```python
from build123d import *

# Parameters (mm, degrees)
ENCLOSURE_SHELL_SKETCH_W      = 76
ENCLOSURE_SHELL_SKETCH_H      = 54
ENCLOSURE_SHELL_FEATURE_DEPTH = 32
ENCLOSURE_GAP_SKETCH_W        = 73
ENCLOSURE_GAP_SKETCH_H        = 51
ENCLOSURE_GAP_FEATURE_DEPTH   = 30
CAMERA_CORD_HOLE_SKETCH_W     = 20
CAMERA_CORD_HOLE_SKETCH_H     = 12
CAMERA_CORD_HOLE_DEPTH        = 3
BATTERY_CUT_REACH             = 78
BATTERY_CUT_DIRECTION_2_DEPTH = 1
RIGHT_TAB_FEATURE_SKETCH_W    = 8
RIGHT_TAB_FEATURE_SKETCH_H    = 5
RIGHT_TAB_FEATURE_DEPTH       = 25
LEFT_TAB_FEATURE_SKETCH_W     = 8
LEFT_TAB_FEATURE_SKETCH_H     = 5
LEFT_TAB_FEATURE_DEPTH        = 25
SKETCH1_W                     = 76
SKETCH1_H                     = 54
BOSS_EXTRUDE1_DEPTH           = 20
CUT_EXTRUDE2_START            = -2
SKETCH5_W                     = 72
SKETCH5_H                     = 50
CUT_EXTRUDE2_DEPTH            = 18
SCREW_SHELL_SKETCH_R          = 2.5
SCREW_SHELL_FEATURE_DEPTH     = 1
SKETCH6_W                     = 58
SKETCH6_H                     = 38
CUT_EXTRUDE3_DEPTH            = 2
SCREW_HOLE_SKETCH_R           = 1.6
CUT_EXTRUDE4_DEPTH            = 2
FILLET1_R                     = 3
FILLET2_R                     = 3
FILLET3_R                     = 3
FILLET4_R                     = 3


with BuildPart() as part:
    # Enclosure Shell Sketch → Enclosure Shell Feature (new body)
    with BuildSketch(Plane(origin=(0, 0, 0), x_dir=(1, 0, 0), z_dir=(0, 1, 0))):
        Rectangle(ENCLOSURE_SHELL_SKETCH_W, ENCLOSURE_SHELL_SKETCH_H)
    extrude(amount=ENCLOSURE_SHELL_FEATURE_DEPTH)

    # Enclosure Gap Sketch → Enclosure Gap Feature (cut)
    with BuildSketch(Plane(origin=(0, 32, 0), x_dir=(1, 0, 0), z_dir=(0, 1, 0))):
        Rectangle(ENCLOSURE_GAP_SKETCH_W, ENCLOSURE_GAP_SKETCH_H)
    extrude(amount=-ENCLOSURE_GAP_FEATURE_DEPTH, mode=Mode.SUBTRACT)

    # Camera Cord Hole Sketch → Camera Cord Hole (cut, through all)
    with BuildSketch(Plane(origin=(0, 2, 0), x_dir=(1, 0, 0), z_dir=(0, 1, 0))):
        with Locations((-17.5, -9.5)):
            Rectangle(CAMERA_CORD_HOLE_SKETCH_W, CAMERA_CORD_HOLE_SKETCH_H)
    extrude(amount=-CAMERA_CORD_HOLE_DEPTH, mode=Mode.SUBTRACT)

    # Battery Cut Sketch → Battery Cut (cut, up to next)
    with BuildSketch(Plane.ZY.offset(-38), mode=Mode.PRIVATE) as battery_cut_sk1:
        Polygon((0, 32), (7.492527579, 32), (7.492527579, 26), (-7.5, 26), (-7.5, 32), align=None)
    battery_cut_tool1 = extrude(battery_cut_sk1.sketch, amount=BATTERY_CUT_REACH, mode=Mode.PRIVATE) & part.part
    add(battery_cut_tool1.solids().sort_by_distance((38, 29, -0.003736))[0], mode=Mode.SUBTRACT)

    # Battery Cut Sketch → Battery Cut direction 2 (cut)
    with BuildSketch(Plane.ZY.offset(-38)):
        Polygon((0, 32), (7.492527579, 32), (7.492527579, 26), (-7.5, 26), (-7.5, 32), align=None)
    extrude(amount=-BATTERY_CUT_DIRECTION_2_DEPTH, mode=Mode.SUBTRACT)

    # Right Tab Feature Sketch → Right Tab Feature (add)
    with BuildSketch(Plane(origin=(38, 0, 0), x_dir=(0, 0, -1), z_dir=(1, 0, 0))):
        with Locations((-18, 5.5)):
            Rectangle(RIGHT_TAB_FEATURE_SKETCH_W, RIGHT_TAB_FEATURE_SKETCH_H)
    extrude(amount=RIGHT_TAB_FEATURE_DEPTH)

    # Left Tab Feature Sketch → Left Tab Feature (add)
    with BuildSketch(Plane.ZY.offset(38)):
        with Locations((18, 5.5)):
            Rectangle(LEFT_TAB_FEATURE_SKETCH_W, LEFT_TAB_FEATURE_SKETCH_H)
    extrude(amount=LEFT_TAB_FEATURE_DEPTH)

    # Sketch1 → Boss-Extrude1 (add)
    with BuildSketch(Plane(origin=(0, 2, 0), x_dir=(1, 0, 0), z_dir=(0, 1, 0))):
        Rectangle(SKETCH1_W, SKETCH1_H)
    extrude(amount=BOSS_EXTRUDE1_DEPTH)

    # Sketch5 → Cut-Extrude2 (cut)
    with BuildSketch(Plane(origin=(0, 0, 0), x_dir=(-1, 0, 0), z_dir=(0, -1, 0)).offset(CUT_EXTRUDE2_START)):
        Rectangle(SKETCH5_W, SKETCH5_H)
    extrude(amount=-CUT_EXTRUDE2_DEPTH, mode=Mode.SUBTRACT)

    # Screw Shell Sketch → Screw Shell Feature (add)
    with BuildSketch(Plane(origin=(0, 22, 0), x_dir=(1, 0, 0), z_dir=(0, 1, 0))):
        with Locations((-30.088214765, 20.515946978)):
            Circle(SCREW_SHELL_SKETCH_R)
        with Locations((-32.1, -21.5)):
            Circle(SCREW_SHELL_SKETCH_R)
        with Locations((32.1, 21.5)):
            Circle(SCREW_SHELL_SKETCH_R)
        with Locations((30.088214765, -20.515946978)):
            Circle(SCREW_SHELL_SKETCH_R)
    extrude(amount=-SCREW_SHELL_FEATURE_DEPTH)

    # Sketch6 → Cut-Extrude3 (cut)
    with BuildSketch(Plane(origin=(0, 22, 0), x_dir=(1, 0, 0), z_dir=(0, 1, 0))):
        Rectangle(SKETCH6_W, SKETCH6_H)
    extrude(amount=-CUT_EXTRUDE3_DEPTH, mode=Mode.SUBTRACT)

    # Screw Hole Sketch → Cut-Extrude4 (cut)
    with BuildSketch(Plane(origin=(0, 22, 0), x_dir=(1, 0, 0), z_dir=(0, 1, 0))):
        with Locations((-31.096, 20.5)):
            Circle(SCREW_HOLE_SKETCH_R)
        with Locations((-31.1, -20.5)):
            Circle(SCREW_HOLE_SKETCH_R)
        with Locations((31.096, -20.5)):
            Circle(SCREW_HOLE_SKETCH_R)
        with Locations((31.1, 20.5)):
            Circle(SCREW_HOLE_SKETCH_R)
    extrude(amount=-CUT_EXTRUDE4_DEPTH, mode=Mode.SUBTRACT)

    # Fillet1
    fillet1_edges = [part.edges().sort_by_distance(p)[0] for p in [
        (-29, 21, -19),
    ]]
    fillet(fillet1_edges, radius=FILLET1_R)

    # Fillet2
    fillet2_edges = [part.edges().sort_by_distance(p)[0] for p in [
        (29, 21, -19),
    ]]
    fillet(fillet2_edges, radius=FILLET2_R)

    # Fillet3
    fillet3_edges = [part.edges().sort_by_distance(p)[0] for p in [
        (29, 21, 19),
    ]]
    fillet(fillet3_edges, radius=FILLET3_R)

    # Fillet4
    fillet4_edges = [part.edges().sort_by_distance(p)[0] for p in [
        (-29, 21, 19),
    ]]
    fillet(fillet4_edges, radius=FILLET4_R)


solid = part.part
```
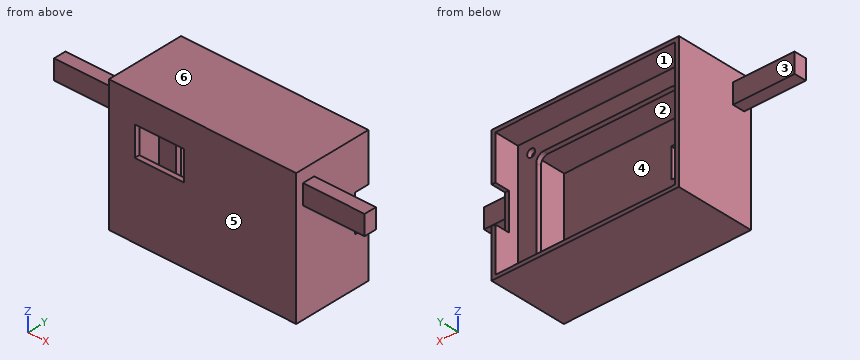
Part model, mm, in its own coordinate system. Face numbers are marked on the shaded views. A direction names the side the tool comes from. Coordinates: 2 decimals unless noted, no trailing zeros. Order: outer loops, then holes, each group sorted by start corner. A loop starts at its lowest first (then second) coordinate and runs counter-clockwise, first axis right, second up. Notation, with made-up numbers: (38.25, 12) -> (72.25, 12) arc R12 cw to (72.25, 26) -> close; hole circle Ø5 at (-16, 43). An arc over 180 degrees is marked (long way). Put each result on its own line as item: value. Start each with the question number.
(1) Band-saw the part on B-B (z = 20.5). Give the cut face in (x, y), then the cut area to 3 significant figures.
(2) Band-saw the part on D-D (y = 24.5). Give the cut face in (x, z), then the cut area to 3 significant figures.
(3) Band-saw the part on C-C (y = 9.5). Give the cut face in (x, z), then the cut area to 3 significant figures.
(4) Band-saw the part on A-A (x = -31.1). Give the cut face in (y, z).
(5) Which spindle directions (+Z, -Z, +X, -X, +Y, -Y) get a long thin tool onto all of the face, cutting with end or side? Do the marked faces 1, 2 and 3. Say none if no direction does.
(6) Pin check, flat tips, straight feed: pin 1 Ø2 at (y, z) = (0.5, 10.5) entering from +X; pin 2 Ø3.5 at (x, z) = (31.1, -20.5) entering from +Y; pin 3 Ø2 at (x, z) = (0.5, 6) entering from +Y. Stop position of each tip, or through.
(7) Mould opens along Z. For the marked faces 4, 5 and 6 say: pulls with the +Z half, pulls with the -Z half, needs draft (parallel to the pull), parting line crosses it, or undercut.
(8) Probe line 1 along X through (y, z) = (20.9, -20.5); line 2 along X through (y, z) = (7.5, 19.5); line 3 along X through (y, z) = (21, 20). List the from-to ranges inside material, lowest first. Write a range as [from, to].
Determined:
1. outline: (-63, 3) -> (-38, 3) -> (-38, 0) -> (38, 0) -> (38, 3) -> (63, 3) -> (63, 8) -> (38, 8) -> (38, 32) -> (36.5, 32) -> (36.5, 22) -> (32.7, 22) -> (32.7, 20) -> (36, 20) -> (36, 2) -> (-36, 2) -> (-36, 20) -> (-32.7, 20) -> (-32.7, 22) -> (-36.5, 22) -> (-36.5, 32) -> (-38, 32) -> (-38, 8) -> (-63, 8) -> close; (-29.5, 20) -> (29.5, 20) -> (29.5, 22) -> (-29.5, 22) -> close
1. area: 643 mm²
2. outline: (-38, -27) -> (38, -27) -> (38, 27) -> (-38, 27) -> close; hole (-36.5, -25.5) -> (36.5, -25.5) -> (36.5, 25.5) -> (-36.5, 25.5) -> close
2. area: 381 mm²
3. outline: (-38, -27) -> (38, -27) -> (38, 27) -> (-38, 27) -> close; hole (-36, -25) -> (36, -25) -> (36, 25) -> (-36, 25) -> close
3. area: 504 mm²
4. outline: (0, -27) -> (32, -27) -> (32, -25.5) -> (22, -25.5) -> (22, -22.1) -> (20, -22.1) -> (20, -25) -> (2, -25) -> (2, 25) -> (20, 25) -> (20, 22.1) -> (22, 22.1) -> (22, 25.5) -> (32, 25.5) -> (32, 27) -> (0, 27) -> close; (20, -18.9) -> (22, -18.9) -> (22, 18.9) -> (20, 18.9) -> close
5. face 1: +Y
5. face 2: none
5. face 3: +Z, -Z, -X, +Y
6. pin 1: stops at x = 38
6. pin 2: stops at y = 22
6. pin 3: stops at y = 2
7. face 4: undercut
7. face 5: needs draft
7. face 6: pulls with the +Z half
8. line 1: x = [-38, -32.7], [-29.5, 29.5], [32.7, 38]
8. line 2: x = [-63, -36], [36, 63]
8. line 3: x = [-38, -32.62], [-29.58, 29.58], [32.62, 38]
